Check sheet for the drawn part. Datum: minimum x, y, z corner. Units: mm. Round coordinates to 2 decimals unless told otherwise and drop trailing zeros. Loops run counter-clockwise (first coordinate to the right, second up) from the corner with the lowest first, then second, coordinate; pieces in that order, holes last.
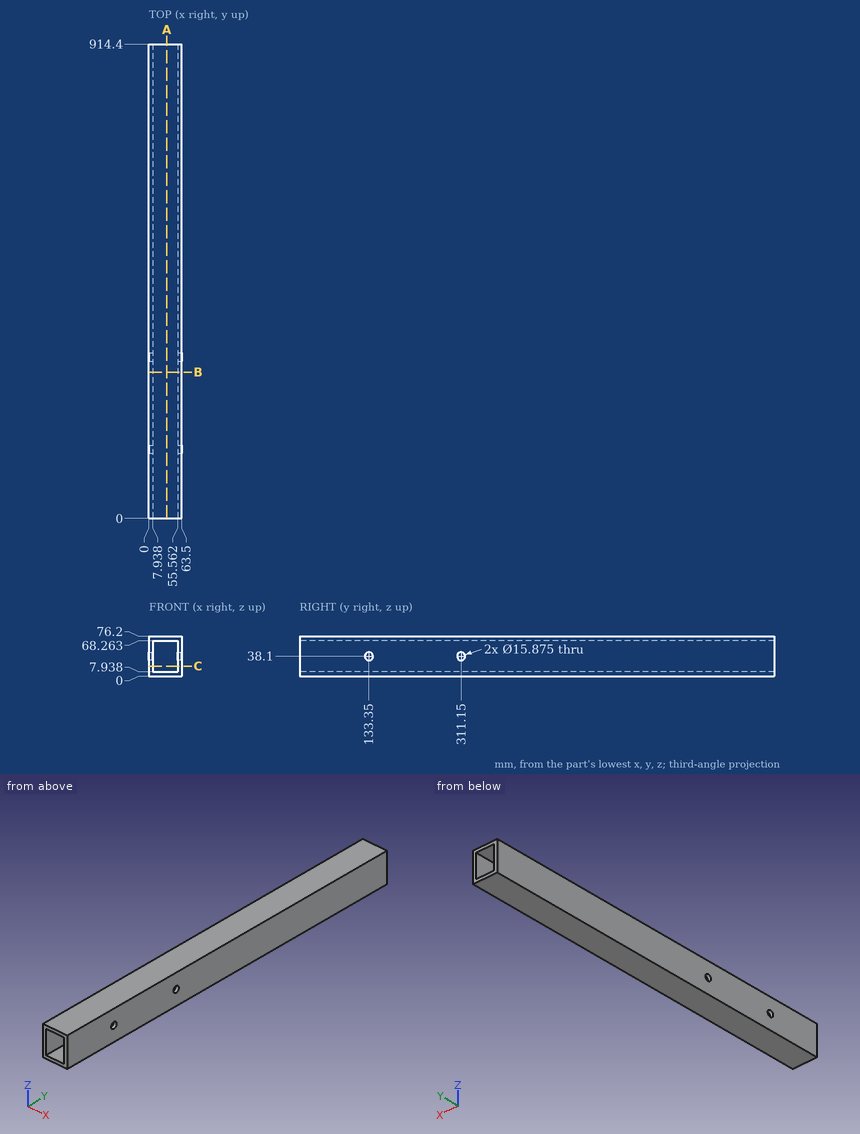
1) Sectioned sample at C-C, the plane z = 19. Record the cut outline in (x, y).
Report:
outline: (0, 0) - (7.94, 0) - (7.94, 914.4) - (0, 914.4) - close; (55.56, 0) - (63.5, 0) - (63.5, 914.4) - (55.56, 914.4) - close
2) Sectioned sample at A-A, the plane x = 35. Record the cut outline in (y, z).
Report:
outline: (0, 0) - (914.4, 0) - (914.4, 7.94) - (0, 7.94) - close; (0, 68.26) - (914.4, 68.26) - (914.4, 76.2) - (0, 76.2) - close
3) Gauge pin test, flat end, axial feed: pin 1 (9.5 mm diameter, centred on y = 311.15, z = 38.1, fed in from +X). Record the tip position at first contact, or that the pin passes through.
Report:
pin 1: passes through
4) Sectioned sample at B-B, the plane y = 282. Record the cut outline in (x, z), then the cut area to 3 significant figures.
Report:
outline: (0, 0) - (63.5, 0) - (63.5, 76.2) - (0, 76.2) - close; hole (7.94, 7.94) - (55.56, 7.94) - (55.56, 68.26) - (7.94, 68.26) - close
area: 1,970 mm2
5) Scan lines: line 1 along Y through (x, z) = (60, 38.1); line 2 along Y through (x, z) = (58, 36.5) (1 decimal); line 3 along X through (y, z) = (394, 64). Record each from-to range of solid material in increasing order.
Report:
line 1: y = 0 to 125.41, 141.29 to 303.21, 319.09 to 914.4
line 2: y = 0 to 125.6, 141.1 to 303.4, 318.9 to 914.4
line 3: x = 0 to 7.94, 55.56 to 63.5
